from build123d import *
from build123d.topology import SkipClean

# Parameters (mm, degrees)
SKETCH1_R                = 3.5
SKETCH1_R_2              = 2.45
HOLE_DEPTH               = 5.2
SKETCH2_W                = 2.5
SKETCH2_H                = 4.5
BOSS_EXTRUDE2_DEPTH      = 5.2
SKETCH3_W                = 4.8
SKETCH3_H                = 9.8
BOSS_EXTRUDE3_DEPTH      = 19
LEVER_ARM_DEPTH          = 5.2
BOSS_EXTRUDE4_DEPTH      = 2.2
BOSS_EXTRUDE4_DEPTH_BACK = 7.4
SKETCH6_R                = 3.5
SKETCH6_R_2              = 2.45
SCALE1_SCALE             = 0.8


with BuildPart() as part:
    # Sketch1 → hole (new body)
    with BuildSketch(Plane(origin=(0, 0, 0), x_dir=(1, 0, 0), z_dir=(0, 1, 0))):
        with Locations(Location((0, 0, 0), (0, 0, 270))):
            Circle(SKETCH1_R)
        with Locations(Location((0, 0, 0), (0, 0, 270))):
            Circle(SKETCH1_R_2, mode=Mode.SUBTRACT)
    extrude(amount=HOLE_DEPTH)

    # Sketch2 → Boss-Extrude2 (add)
    with BuildSketch(Plane.XZ):
        with Locations((0, -5.75)):
            Rectangle(SKETCH2_W, SKETCH2_H)
        with BuildLine():
            ThreePointArc((1.25, -3.269174208), (0.635566784, -3.441809824), (0, -3.5))
            Line((0, -3.5), (1.25, -3.5))
            Line((1.25, -3.5), (1.25, -3.269174208))
        make_face()
        with BuildLine():
            Line((-1.25, -3.269174208), (-1.25, -3.5))
            Line((-1.25, -3.5), (0, -3.5))
            ThreePointArc((0, -3.5), (-0.635566784, -3.441809824), (-1.25, -3.269174208))
        make_face()
    extrude(amount=-BOSS_EXTRUDE2_DEPTH)

    # Sketch3 → Boss-Extrude3 (add)
    with BuildSketch(Plane(origin=(0, 0, -8), x_dir=(-1, 0, 0), z_dir=(0, 0, -1))):
        with Locations((0, 2.6)):
            Rectangle(SKETCH3_W, SKETCH3_H)
    extrude(amount=BOSS_EXTRUDE3_DEPTH)

    # Sketch5 → lever arm (add)
    with BuildSketch(Plane.XZ):
        Polygon((-18.75, -6.884587104), (-1.25, -6.884587104), (-1.25, -4.384587104), (-16.25, -4.384587104), (-18.75, -4.384587104), align=None)
        with BuildLine():
            ThreePointArc((-21.25, -4.384587104), (-20.517766953, -6.152354057), (-18.75, -6.884587104))
            Line((-18.75, -6.884587104), (-18.75, -4.384587104))
            Line((-18.75, -4.384587104), (-21.25, -4.384587104))
        make_face()
        with BuildLine():
            Line((-18.75, -1.884587104), (-18.75, -4.384587104))
            Line((-18.75, -4.384587104), (-16.25, -4.384587104))
            ThreePointArc((-16.25, -4.384587104), (-18.017766953, -3.652354057), (-18.75, -1.884587104))
        make_face()
        Polygon((-21.25, -4.384587104), (-18.75, -4.384587104), (-18.75, -1.884587104), (-18.75, 5.615412896), (-21.25, 5.615412896), align=None)
    extrude(amount=-LEVER_ARM_DEPTH)

    # Sketch6 → Boss-Extrude4 (add, two sides: drawn at the far end of the back side and taken through both)
    with SkipClean():  # the faces are left unmerged after this step: merging them gives an invalid solid
        with BuildSketch(Plane.XZ.offset(-BOSS_EXTRUDE4_DEPTH_BACK)):
            with Locations(Location((0, 0, 0), (0, 0, 270))):
                Circle(SKETCH6_R)
            with Locations(Location((0, 0, 0), (0, 0, 270))):
                Circle(SKETCH6_R_2, mode=Mode.SUBTRACT)
        extrude(amount=BOSS_EXTRUDE4_DEPTH + BOSS_EXTRUDE4_DEPTH_BACK)
    add(part.part.scale(1), mode=Mode.REPLACE)  # the faces are merged on a copy


with BuildPart() as part_1:
    # Scale1: scaled about (-3.5957974, 2.6, -11.326296727)
    add(part.part.scale(SCALE1_SCALE).moved(Location((-0.71915948, 0.52, -2.265259345))))


solid = part_1.part
Read the model definition and answer for the solid it produces. Units are mm, in the model's axes. A direction names the side the tool comes from. Coordinates: 2 decimals unless noted, no trailing zeros. Order: outer loops, then holes, each group sorted by start corner. A loop starts at its lowest first (then second) coordinate and runs counter-clockwise, first axis right, second up. Notation, with made-up numbers: M -9,88 L 2,88 A3 cw 2,92 Z; hole C 5,78 d5. An arc over 180 degrees is marked long. Put each result on its own line as item: value. Start each with the question number.
Item 1: Section D-D, the plane y = 2.75 is taken. Determine the outline of the cut face in (x, z).
Item 2: Consider probe 1 along Z at (x, y) = (-2.5, 4.75); probe 2 along Y at (x, z) = (-2.5, -3.75); probe 3 along Z at (x, y) = (-15.25, 4.25). Determine where each line is inside the solid, lowest interval first. Write a range as [from, to].
Item 3: Given pin 1 Ø1 at (x, y) = (-8, 2) entering from +Z; pin 2 Ø1 at (y, z) = (5, -7) entering from -X; pin 3 Ø4 at (y, z) = (3.5, -7) entering from +X, each flat-ended and moving along its own axis, determine where each tip first touches the part or whether it passes through.
Item 4: Section B-B, the plane y = 0.25 is taken. Determine the outline of the cut face in (x, z).
Item 5: For faces 1 (the face through (-2.639, 3, -16)), 2 (the face through (-1, -1.24, 0)), 3 (the face through (-1, 6.44, 0)), 4 (the face through (-1.719, 2.6, -5.3)), 5 (the face through (-15.12, 2.57, -5.2)), determine the directions among +Z, -Z, +X, -X, +Y, -Y from which every point of the face is accessible in a straight line to the end or side of a thin tool.
Item 6: The mould has two halves that part along X. Classify faces 6 (the face through (-1.719, 3, -8)), 7 (the face through (-8, 3, -5.773)), 8 (the face through (0.281, 3, -7)): +X half, -X half, draft (parallel to the pull), parting line (faces both ways), or undercut.
Item 7: Section A-A, the plane z = -5.5 is taken. Determine the outline of the cut face in (x, y), plus the area to 3 significant figures.
Item 8: Section C-C, the plane x = -1 is taken. Determine the outline of the cut face in (y, z), plus the area to 3 significant figures.
Computed:
1. outline: M -17.72,-5.77 A2 ccw -15.72,-7.77 L -1.72,-7.77 L -1.72,-8.67 L -2.64,-8.67 L -2.64,-23.87 L 1.2,-23.87 L 1.2,-8.67 L 0.28,-8.67 L 0.28,-4.88 A2.8 ccw long -1.72,-4.88 L -1.72,-5.77 L -13.72,-5.77 A2 cw -15.72,-3.77 L -15.72,2.23 L -17.72,2.23 Z; hole C -0.72,-2.27 d3.92
2. probe 1: z = [-23.87, -8.67], [-4.43, -3.08], [-1.45, -0.1]
2. probe 2: y = [-1.24, 6.44]
2. probe 3: z = [-7.77, -5.06]
3. pin 1: stops at z = -5.77
3. pin 2: stops at x = -17.53
3. pin 3: stops at x = 1.2
4. outline: C -0.72,-2.27 d5.6; M -2.64,-23.87 L 1.2,-23.87 L 1.2,-8.67 L -2.64,-8.67 Z; hole C -0.72,-2.27 d3.92
5. face 1: -Z, -X, +Y, -Y
5. face 2: +Z, +X, -X, -Y
5. face 3: +Z, +X, -X, +Y
5. face 4: +Y, -Y
5. face 5: +Z, +Y, -Y
6. face 6: -X half
6. face 7: undercut
6. face 8: +X half
7. outline: M -17.72,0.52 L -14.73,0.52 L -14.73,4.68 L -17.72,4.68 Z; M -1.72,0.52 L 0.28,0.52 L 0.28,4.68 L -1.72,4.68 Z
7. area: 20.8 mm2
8. outline: M -1.32,-23.87 L 6.52,-23.87 L 6.52,-8.67 L 4.68,-8.67 L 4.68,-5.05 L 6.44,-5.05 L 6.44,-4.21 L -1.24,-4.21 L -1.24,-5.05 L 0.52,-5.05 L 0.52,-8.67 L -1.32,-8.67 Z; M -1.24,-0.33 L 6.44,-0.33 L 6.44,0.52 L -1.24,0.52 Z
8. area: 147 mm2
